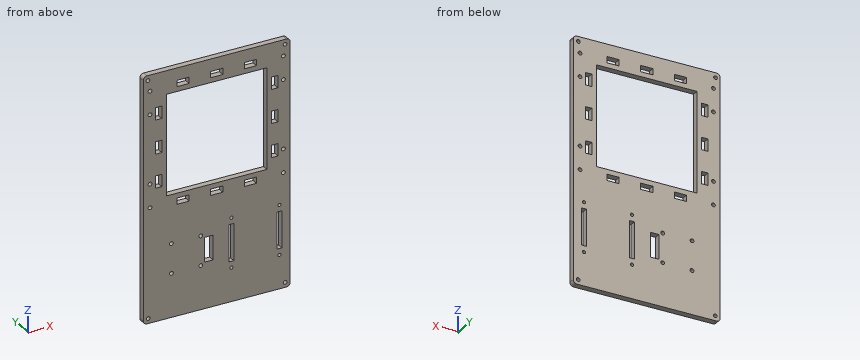
from build123d import *

# Parameters (mm, degrees)
SKETCH1_W           = 120
SKETCH1_H           = 200
SKETCH1_R           = 1.5
BOSS_EXTRUDE1_DEPTH = 5
CUT_EXTRUDE1_REACH  = 118.726
SKETCH4_W           = 5.1
SKETCH4_H           = 10
SKETCH4_W_2         = 10
SKETCH4_H_2         = 5.1
SKETCH4_W_3         = 82
SKETCH4_H_3         = 82
SKETCH5_R           = 1.55
SKETCH5_W           = 7.015063312
SKETCH5_H           = 20
CUT_EXTRUDE3_DEPTH  = 117.726175299
SKETCH6_W           = 4
SKETCH6_H           = 30
SKETCH6_R           = 1.3
CUT_EXTRUDE5_DEPTH  = 10
SKETCH7_R           = 1.55
CUT_EXTRUDE6_DEPTH  = 117.726175299
FILLET1_R           = 3


with BuildPart() as part:
    # Sketch1 → Boss-Extrude1 (new body)
    with BuildSketch(Plane(origin=(0, 0, 0), x_dir=(1, 0, 0), z_dir=(0, 1, 0))):
        Rectangle(SKETCH1_W, SKETCH1_H)
        with Locations(Location((-56, 96, 0), (0, 0, 270))):
            Circle(SKETCH1_R, mode=Mode.SUBTRACT)
        with Locations(Location((56, 96, 0), (0, 0, 270))):
            Circle(SKETCH1_R, mode=Mode.SUBTRACT)
        with Locations(Location((55.822222222, -96, 0), (0, 0, 270))):
            Circle(SKETCH1_R, mode=Mode.SUBTRACT)
        with Locations(Location((-56.177777778, -96, 0), (0, 0, 270))):
            Circle(SKETCH1_R, mode=Mode.SUBTRACT)
    extrude(amount=BOSS_EXTRUDE1_DEPTH)

    # Sketch4 → Cut-Extrude1 (cut, up to next)
    with BuildSketch(Plane(origin=(0, 5, 0), x_dir=(1, 0, 0), z_dir=(0, 1, 0)), mode=Mode.PRIVATE) as cut_extrude1_sk1:
        with Locations((-47.45, -12.5)):
            Rectangle(SKETCH4_W, SKETCH4_H)
    cut_extrude1_tool1 = extrude(cut_extrude1_sk1.sketch, amount=-CUT_EXTRUDE1_REACH, mode=Mode.PRIVATE) & part.part
    # Sketch4 → Cut-Extrude1 (cut, up to next)
    with BuildSketch(Plane(origin=(0, 5, 0), x_dir=(1, 0, 0), z_dir=(0, 1, 0)), mode=Mode.PRIVATE) as cut_extrude1_sk2:
        with Locations((-47.45, -67.5)):
            Rectangle(SKETCH4_W, SKETCH4_H)
    cut_extrude1_tool2 = extrude(cut_extrude1_sk2.sketch, amount=-CUT_EXTRUDE1_REACH, mode=Mode.PRIVATE) & part.part
    # Sketch4 → Cut-Extrude1 (cut, up to next)
    with BuildSketch(Plane(origin=(0, 5, 0), x_dir=(1, 0, 0), z_dir=(0, 1, 0)), mode=Mode.PRIVATE) as cut_extrude1_sk3:
        with Locations((-47.45, -40)):
            Rectangle(SKETCH4_W, SKETCH4_H)
    cut_extrude1_tool3 = extrude(cut_extrude1_sk3.sketch, amount=-CUT_EXTRUDE1_REACH, mode=Mode.PRIVATE) & part.part
    # Sketch4 → Cut-Extrude1 (cut, up to next)
    with BuildSketch(Plane(origin=(0, 5, 0), x_dir=(1, 0, 0), z_dir=(0, 1, 0)), mode=Mode.PRIVATE) as cut_extrude1_sk4:
        with Locations((-27.5, 7.45)):
            Rectangle(SKETCH4_W_2, SKETCH4_H_2)
    cut_extrude1_tool4 = extrude(cut_extrude1_sk4.sketch, amount=-CUT_EXTRUDE1_REACH, mode=Mode.PRIVATE) & part.part
    # Sketch4 → Cut-Extrude1 (cut, up to next)
    with BuildSketch(Plane(origin=(0, 5, 0), x_dir=(1, 0, 0), z_dir=(0, 1, 0)), mode=Mode.PRIVATE) as cut_extrude1_sk5:
        with Locations((0, 7.45)):
            Rectangle(SKETCH4_W_2, SKETCH4_H_2)
    cut_extrude1_tool5 = extrude(cut_extrude1_sk5.sketch, amount=-CUT_EXTRUDE1_REACH, mode=Mode.PRIVATE) & part.part
    # Sketch4 → Cut-Extrude1 (cut, up to next)
    with BuildSketch(Plane(origin=(0, 5, 0), x_dir=(1, 0, 0), z_dir=(0, 1, 0)), mode=Mode.PRIVATE) as cut_extrude1_sk6:
        with Locations((27.5, 7.45)):
            Rectangle(SKETCH4_W_2, SKETCH4_H_2)
    cut_extrude1_tool6 = extrude(cut_extrude1_sk6.sketch, amount=-CUT_EXTRUDE1_REACH, mode=Mode.PRIVATE) & part.part
    # Sketch4 → Cut-Extrude1 (cut, up to next)
    with BuildSketch(Plane(origin=(0, 5, 0), x_dir=(1, 0, 0), z_dir=(0, 1, 0)), mode=Mode.PRIVATE) as cut_extrude1_sk7:
        with Locations((47.45, -12.5)):
            Rectangle(SKETCH4_W, SKETCH4_H)
    cut_extrude1_tool7 = extrude(cut_extrude1_sk7.sketch, amount=-CUT_EXTRUDE1_REACH, mode=Mode.PRIVATE) & part.part
    # Sketch4 → Cut-Extrude1 (cut, up to next)
    with BuildSketch(Plane(origin=(0, 5, 0), x_dir=(1, 0, 0), z_dir=(0, 1, 0)), mode=Mode.PRIVATE) as cut_extrude1_sk8:
        with Locations((47.45, -40)):
            Rectangle(SKETCH4_W, SKETCH4_H)
    cut_extrude1_tool8 = extrude(cut_extrude1_sk8.sketch, amount=-CUT_EXTRUDE1_REACH, mode=Mode.PRIVATE) & part.part
    # Sketch4 → Cut-Extrude1 (cut, up to next)
    with BuildSketch(Plane(origin=(0, 5, 0), x_dir=(1, 0, 0), z_dir=(0, 1, 0)), mode=Mode.PRIVATE) as cut_extrude1_sk9:
        with Locations((47.45, -67.5)):
            Rectangle(SKETCH4_W, SKETCH4_H)
    cut_extrude1_tool9 = extrude(cut_extrude1_sk9.sketch, amount=-CUT_EXTRUDE1_REACH, mode=Mode.PRIVATE) & part.part
    # Sketch4 → Cut-Extrude1 (cut, up to next)
    with BuildSketch(Plane(origin=(0, 5, 0), x_dir=(1, 0, 0), z_dir=(0, 1, 0)), mode=Mode.PRIVATE) as cut_extrude1_sk10:
        with Locations((0, -87.45)):
            Rectangle(SKETCH4_W_2, SKETCH4_H_2)
    cut_extrude1_tool10 = extrude(cut_extrude1_sk10.sketch, amount=-CUT_EXTRUDE1_REACH, mode=Mode.PRIVATE) & part.part
    # Sketch4 → Cut-Extrude1 (cut, up to next)
    with BuildSketch(Plane(origin=(0, 5, 0), x_dir=(1, 0, 0), z_dir=(0, 1, 0)), mode=Mode.PRIVATE) as cut_extrude1_sk11:
        with Locations((-27.5, -87.45)):
            Rectangle(SKETCH4_W_2, SKETCH4_H_2)
    cut_extrude1_tool11 = extrude(cut_extrude1_sk11.sketch, amount=-CUT_EXTRUDE1_REACH, mode=Mode.PRIVATE) & part.part
    # Sketch4 → Cut-Extrude1 (cut, up to next)
    with BuildSketch(Plane(origin=(0, 5, 0), x_dir=(1, 0, 0), z_dir=(0, 1, 0)), mode=Mode.PRIVATE) as cut_extrude1_sk12:
        with Locations((27.5, -87.45)):
            Rectangle(SKETCH4_W_2, SKETCH4_H_2)
    cut_extrude1_tool12 = extrude(cut_extrude1_sk12.sketch, amount=-CUT_EXTRUDE1_REACH, mode=Mode.PRIVATE) & part.part
    # Sketch4 → Cut-Extrude1 (cut, up to next)
    with BuildSketch(Plane(origin=(0, 5, 0), x_dir=(1, 0, 0), z_dir=(0, 1, 0)), mode=Mode.PRIVATE) as cut_extrude1_sk13:
        with Locations((0, -40)):
            Rectangle(SKETCH4_W_3, SKETCH4_H_3)
    cut_extrude1_tool13 = extrude(cut_extrude1_sk13.sketch, amount=-CUT_EXTRUDE1_REACH, mode=Mode.PRIVATE) & part.part
    add(cut_extrude1_tool1.solids().sort_by_distance((-47.45, 5, 12.5))[0], mode=Mode.SUBTRACT)
    add(cut_extrude1_tool2.solids().sort_by_distance((-47.45, 5, 67.5))[0], mode=Mode.SUBTRACT)
    add(cut_extrude1_tool3.solids().sort_by_distance((-47.45, 5, 40))[0], mode=Mode.SUBTRACT)
    add(cut_extrude1_tool4.solids().sort_by_distance((-27.5, 5, -7.45))[0], mode=Mode.SUBTRACT)
    add(cut_extrude1_tool5.solids().sort_by_distance((0, 5, -7.45))[0], mode=Mode.SUBTRACT)
    add(cut_extrude1_tool6.solids().sort_by_distance((27.5, 5, -7.45))[0], mode=Mode.SUBTRACT)
    add(cut_extrude1_tool7.solids().sort_by_distance((47.45, 5, 12.5))[0], mode=Mode.SUBTRACT)
    add(cut_extrude1_tool8.solids().sort_by_distance((47.45, 5, 40))[0], mode=Mode.SUBTRACT)
    add(cut_extrude1_tool9.solids().sort_by_distance((47.45, 5, 67.5))[0], mode=Mode.SUBTRACT)
    add(cut_extrude1_tool10.solids().sort_by_distance((0, 5, 87.45))[0], mode=Mode.SUBTRACT)
    add(cut_extrude1_tool11.solids().sort_by_distance((-27.5, 5, 87.45))[0], mode=Mode.SUBTRACT)
    add(cut_extrude1_tool12.solids().sort_by_distance((27.5, 5, 87.45))[0], mode=Mode.SUBTRACT)
    add(cut_extrude1_tool13.solids().sort_by_distance((0, 5, 40))[0], mode=Mode.SUBTRACT)

    # Sketch5 → Cut-Extrude3 (cut, through all)
    with BuildSketch(Plane(origin=(0, 5, 0), x_dir=(1, 0, 0), z_dir=(0, 1, 0))):
        with Locations(Location((-37, 64.5, 0), (0, 0, 270))):
            Circle(SKETCH5_R)
        with Locations(Location((-13, 64.5, 0), (0, 0, 270))):
            Circle(SKETCH5_R)
        with Locations(Location((-13, 40.5, 0), (0, 0, 270))):
            Circle(SKETCH5_R)
        with Locations(Location((-37, 40.5, 0), (0, 0, 270))):
            Circle(SKETCH5_R)
        with Locations((-6.492468344, 52.5)):
            Rectangle(SKETCH5_W, SKETCH5_H)
    extrude(amount=-CUT_EXTRUDE3_DEPTH, mode=Mode.SUBTRACT)

    # Sketch6 → Cut-Extrude5 (cut)
    with BuildSketch(Plane(origin=(0, 5, 0), x_dir=(1, 0, 0), z_dir=(0, 1, 0))):
        with Locations((12, 52.5)):
            Rectangle(SKETCH6_W, SKETCH6_H)
        with Locations((51.25, 52.5)):
            Rectangle(SKETCH6_W, SKETCH6_H)
        with Locations(Location((51.25, 72.625, 0), (0, 0, 270))):
            Circle(SKETCH6_R)
        with Locations(Location((12, 72.625, 0), (0, 0, 270))):
            Circle(SKETCH6_R)
        with Locations(Location((12, 32.375, 0), (0, 0, 270))):
            Circle(SKETCH6_R)
        with Locations(Location((51.25, 32.375, 0), (0, 0, 270))):
            Circle(SKETCH6_R)
    extrude(amount=-CUT_EXTRUDE5_DEPTH, mode=Mode.SUBTRACT)

    # Sketch7 → Cut-Extrude6 (cut, through all)
    with BuildSketch(Plane(origin=(0, 5, 0), x_dir=(1, 0, 0), z_dir=(0, 1, 0))):
        with Locations(Location((-54.5, 7, 0), (0, 0, 270))):
            Circle(SKETCH7_R)
        with Locations(Location((-54.5, -12, 0), (0, 0, 270))):
            Circle(SKETCH7_R)
        with Locations(Location((-54.5, -68, 0), (0, 0, 90))):
            Circle(SKETCH7_R)
        with Locations(Location((-54.5, -87, 0), (0, 0, 90))):
            Circle(SKETCH7_R)
        with Locations(Location((54.5, -12, 0), (0, 0, 90))):
            Circle(SKETCH7_R)
        with Locations(Location((54.5, 7, 0), (0, 0, 90))):
            Circle(SKETCH7_R)
        with Locations(Location((54.5, -87, 0), (0, 0, 270))):
            Circle(SKETCH7_R)
        with Locations(Location((54.5, -68, 0), (0, 0, 270))):
            Circle(SKETCH7_R)
    extrude(amount=-CUT_EXTRUDE6_DEPTH, mode=Mode.SUBTRACT)

    # Fillet1
    fillet1_edges = [part.edges().sort_by_distance(p)[0] for p in [
        (-60, 2.5, 100),
        (-60, 2.5, -100),
        (60, 2.5, -100),
        (60, 2.5, 100),
    ]]
    fillet(fillet1_edges, radius=FILLET1_R)


solid = part.part
Can you work these out from the model? Positions are in its coordinate system, mm. Give positions to 0.01 mm unless a question says otherwise; leave off trailing zeros. Order: outer loops, then holes, each group sorted by start corner. A loop starts at its lowest first (then second) coordinate and runs counter-clockwise, first axis right, second up. Notation, with made-up numbers: M -0.5,-17.5 L 51.5,-17.5 A8 ccw 51.5,-2.5 Z; hole C 65.25,-19.75 d7. An arc over 180 degrees is marked long. Use one line per item in the form item = value. Start each with the question number.
Item 1: If we section it at B-B (y = 2): State how many separate pieces and enclosed holes the cut face has, then the cut area to 3 significant figures.
Item 2: If I drill on line 1 along X through (y, z) = (2.45, 87); line 2 along X through (y, z) = (3.7, -62); line 3 along Z through (x, y) = (-45, 0.2), over which ranges is the centre line in solid material (lowest first)?
Item 3: If we section it at A-A (z = 40.5): Write out the boundary of the cut face in (x, y), then the cut area to 3 significant figures.
Outcome:
q1.separate_pieces = 1
q1.enclosed_holes = 36
q1.area = 16,100 mm2
q2.line_1 = -60 to -56.05, -52.95 to -32.5, -22.5 to -5, 5 to 22.5, 32.5 to 52.95, 56.05 to 60
q2.line_2 = -60 to -10, -2.98 to 10, 14 to 49.25, 53.25 to 60
q2.line_3 = -100 to 7.5, 17.5 to 35, 45 to 62.5, 72.5 to 100
q3.outline = M -60,0 L -50,0 L -50,5 L -60,5 Z; M -44.9,0 L -41,0 L -41,5 L -44.9,5 Z; M 41,0 L 44.9,0 L 44.9,5 L 41,5 Z; M 50,0 L 60,0 L 60,5 L 50,5 Z
q3.area = 139 mm2
